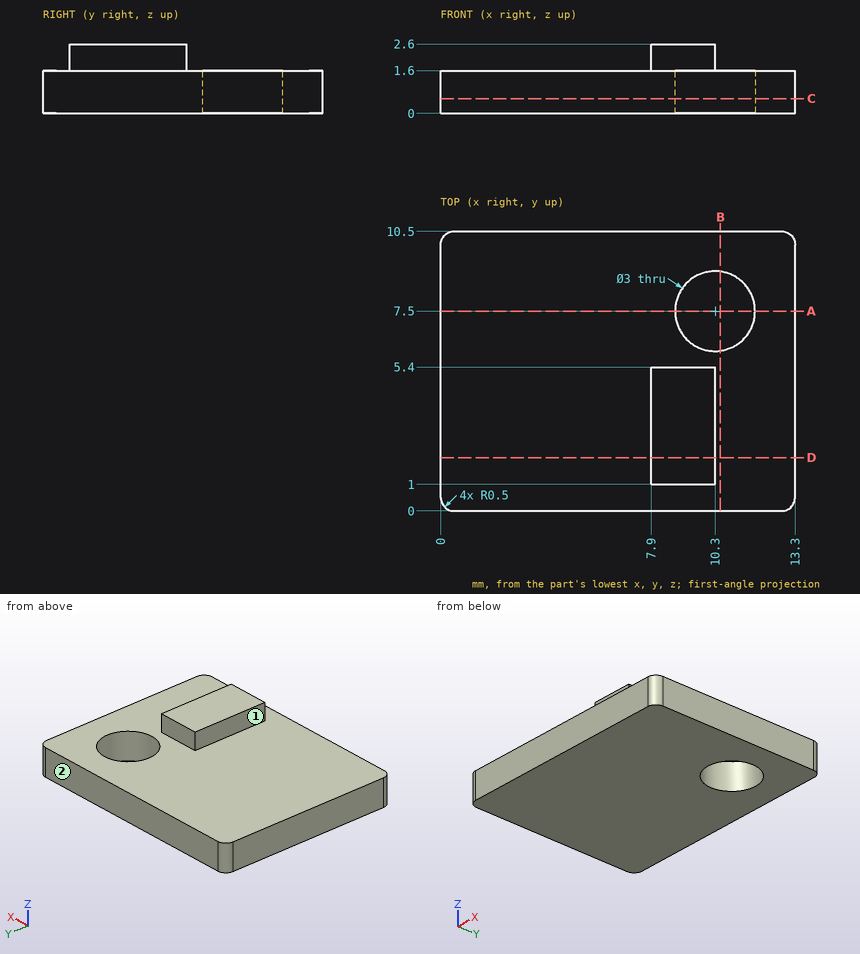
Answer from the drawing. Dimensions are ordinates in mm from the lowest x, y and z of the part. A direction names the side the tool comes from. Round coordinates to 2 decimals unless told otherwise and drop trailing zeros. Order: outer loops, then holes, each group sorted by start corner. A loop starts at its lowest first (then second) coordinate and runs counter-clockwise, first axis right, second up.
1) Flat-ended cylindrical pins translate along their axes: pin 1 (0.5 mm diameter, centred on y = 3, z = 2, fed in from -X); pin 2 (3.5 mm diameter, centred on x = 10.3, y = 7.5, fed in from +Z). Find the tip coordinate at first contact, or state that the pin passes through.
2) Straight lines are drawn through the part: L1, parallel to Y at x = 10.3, z = 0.75; L2, parallel to Z at x = 10.25, y = 5.75; L3, parallel to X at y = 3.5, z = 1.95. For each, find the intervals that lie inside material, in ascending order.
3) For the marked faces 1 and 2, determine the directions among +Z, -Z, +X, -X, +Y, -Y from which every point of the face is accessible in a straight line to the end or side of a thin tool.
4) The part is cut by section D-D on y = 2. Write down the section's boundary in (x, z).
5) The part is cut by section B-B on x = 10.5. Write down the section's boundary in (y, z), plus the area to 3 significant figures.
6) The part is cut by section C-C on z = 0.55. Write down the section's boundary in (x, y).
7) The part is cut by section A-A on y = 7.5. Write down the section's boundary in (x, z).
Resolved:
1. pin 1: stops at x = 7.9
1. pin 2: stops at z = 1.6
2. L1: y = 0 to 6, 9 to 10.5
2. L2: z = 0 to 1.6
2. L3: x = 7.9 to 10.3
3. face 1: +Z, -X, +Y, -Y
3. face 2: +Z, -Z, +X, -X, +Y
4. outline: (0, 0) - (13.3, 0) - (13.3, 1.6) - (10.3, 1.6) - (10.3, 2.6) - (7.9, 2.6) - (7.9, 1.6) - (0, 1.6) - close
5. outline: (0, 0) - (6.01, 0) - (6.01, 1.6) - (0, 1.6) - close; (8.99, 0) - (10.5, 0) - (10.5, 1.6) - (8.99, 1.6) - close
5. area: 12.0 mm2
6. outline: (0, 0.5) arc R0.5 ccw to (0.5, 0) - (12.8, 0) arc R0.5 ccw to (13.3, 0.5) - (13.3, 10) arc R0.5 ccw to (12.8, 10.5) - (0.5, 10.5) arc R0.5 ccw to (0, 10) - close; hole circle Ø3 at (10.3, 7.5)
7. outline: (0, 0) - (8.8, 0) - (8.8, 1.6) - (0, 1.6) - close; (11.8, 0) - (13.3, 0) - (13.3, 1.6) - (11.8, 1.6) - close
